Verification items for the finished model (mm, model axes). Round coordinates to 2 decimals unless told otherwise and drop trailing zeros. Loops run counter-clockwise (first coordinate to the right, second up) from the corner with the lowest first, then second, coordinate; pieces in that order, holes last. Notation, with made-up numbers: (7, -7.5) -> (55, -7.5) arc R10 ccw to (55, 8.5) -> close; hole circle Ø8 at (-1, 57.5). An arc over 180 degrees is marked (long way). Write item = value, one per line.
```python
from build123d import *

# Parameters (mm, degrees)
SKETCH_1_R      = 19.5
EXTRUDE_1_DEPTH = 60
FILLET_1_R      = 10


with BuildPart() as part:
    # 草图1 → 凸台-拉伸1 (new body)
    with BuildSketch(Plane(origin=(0, 0, 0), x_dir=(1, 0, 0), z_dir=(0, 1, 0))):
        Polygon((-22.25, 22.25), (22.25, 22.25), (22.25, -22.25), (22.25, -47.25), (-22.25, -47.25), (-22.25, -22.25), align=None)
        with Locations((0, -22.25)):
            Circle(SKETCH_1_R, mode=Mode.SUBTRACT)
    extrude(amount=EXTRUDE_1_DEPTH)

    # 圆角1
    fillet_1_edges = [part.edges().sort_by_distance(p)[0] for p in [
        (22.25, 30, 47.25),
        (-22.25, 30, 47.25),
        (-22.25, 30, -22.25),
        (22.25, 30, -22.25),
    ]]
    fillet(fillet_1_edges, radius=FILLET_1_R)


solid = part.part
```
(1) Sectioned sample at A-A, the plane x = 0. Record the cut outline in (y, z).
Filled sheet:
outline = (0, -22.25) -> (60, -22.25) -> (60, 2.75) -> (0, 2.75) -> close; (0, 41.75) -> (60, 41.75) -> (60, 47.25) -> (0, 47.25) -> close
(2) Sectioned sample at C-C, the plane z = 22.25. Record the cut outline in (x, y).
Filled sheet:
outline = (-22.25, 0) -> (-19.5, 0) -> (-19.5, 60) -> (-22.25, 60) -> close; (19.5, 0) -> (22.25, 0) -> (22.25, 60) -> (19.5, 60) -> close
(3) Go/stop test with flat-tipped pins: pin 1 Ø8 at (x, z) = (-15.5, 23.5) entering from -Y; pin 2 Ø6 at (x, y) = (-16.5, 31.5) entering from +Z; pin 3 Ø2 at (x, y) = (-14, 54) entering from -Z. Record where each tip stops, or that it passes through.
Filled sheet:
pin_1 = 0
pin_2 = 47.17
pin_3 = -22.22
(4) Draft check along X on faces 1 (the face through (22.25, 30, 13)), 2 (the face through (-10, 0, 4)), 3 (the face through (-2.539, 29.58, 2.916)). Enter one of: released by +X, released by -X, zero draft, split by the parting line, or undercut.
Filled sheet:
face_1 = released by +X
face_2 = zero draft
face_3 = undercut
(5) Sectioned sample at B-B, the plane y = 23.5. Record the cut outline in (x, z).
Filled sheet:
outline = (-22.25, -12.25) arc R10 ccw to (-12.25, -22.25) -> (12.25, -22.25) arc R10 ccw to (22.25, -12.25) -> (22.25, 37.25) arc R10 ccw to (12.25, 47.25) -> (-12.25, 47.25) arc R10 ccw to (-22.25, 37.25) -> close; hole circle Ø39 at (0, 22.25)
(6) Material ranges on probe 1 along Z at (x, y) = (0, 38.5); probe 2 along X at (y, z) = (25, 22.25); probe 3 along Z at (x, y) = (-7.5, 53), recorded low to high. Write a range as from..to.
Filled sheet:
probe_1 = -22.25..2.75, 41.75..47.25
probe_2 = -22.25..-19.5, 19.5..22.25
probe_3 = -22.25..4.25, 40.25..47.25
